Design review of the part built by this model. Coordinates are the model's own, in mm. Coordinates: 2 decimals unless noted, no trailing zeros. Loops run counter-clockwise (first coordinate to the right, second up) from the corner with the lowest first, then second, coordinate; pieces in that order, holes last.
Q1. Add section C-C on z = -18.5. Give the boundary of the cut face in (x, y), and give its area (3 significant figures).
Q2. Add section B-B on y = 0.65. Give the boundary of the cut face in (x, z).
Q3. Add section A-A on x = 1. Give the boundary of the cut face in (y, z), and give its area (3 significant figures).
Q4. For P1, Ø1.2, axis at x = 6, z = -18.5, coming from the +Y side, flat-tipped, find the tip position at first contact; note if it passes through.
Q5. Wall thickness on probe 1 along X at (y, z) = (1.1, -13.5); probe 2 along X at (y, z) = (1.35, -13); probe 3 along X at (y, z) = (1.2, -28): over which ranges is each line inside the solid? List them lowest first.
```python
from build123d import *

# Parameters (mm, degrees)
BOSS_EXTRUDE1_DEPTH = 2
CUT_EXTRUDE2_REACH  = 58.071
SKETCH8_R           = 0.75


with BuildPart() as part:
    # Sketch1 → Boss-Extrude1 (new body)
    with BuildSketch(Plane(origin=(0, 0, 0), x_dir=(1, 0, 0), z_dir=(0, 1, 0))):
        with BuildLine():
            Line((5, 0), (41, 0))
            ThreePointArc((41, 0), (44.535533906, 1.464466094), (46, 5))
            Line((46, 5), (46, 27))
            ThreePointArc((46, 27), (44.535533906, 30.535533906), (41, 32))
            Line((41, 32), (5, 32))
            ThreePointArc((5, 32), (1.464466094, 30.535533906), (0, 27))
            Line((0, 27), (0, 5))
            ThreePointArc((0, 5), (1.464466094, 1.464466094), (5, 0))
        make_face()
    extrude(amount=BOSS_EXTRUDE1_DEPTH)

    # Sketch8 → Cut-Extrude2 (cut, up to next)
    with BuildSketch(Plane(origin=(0, 2, 0), x_dir=(1, 0, 0), z_dir=(0, 1, 0)), mode=Mode.PRIVATE) as cut_extrude2_sk1:
        with Locations(Location((3.5, 16, 0), (0, 0, 270))):
            Circle(SKETCH8_R)
    cut_extrude2_tool1 = extrude(cut_extrude2_sk1.sketch, amount=-CUT_EXTRUDE2_REACH, mode=Mode.PRIVATE) & part.part
    # Sketch8 → Cut-Extrude2 (cut, up to next)
    with BuildSketch(Plane(origin=(0, 2, 0), x_dir=(1, 0, 0), z_dir=(0, 1, 0)), mode=Mode.PRIVATE) as cut_extrude2_sk2:
        with Locations(Location((6, 18.5, 0), (0, 0, 270))):
            Circle(SKETCH8_R)
    cut_extrude2_tool2 = extrude(cut_extrude2_sk2.sketch, amount=-CUT_EXTRUDE2_REACH, mode=Mode.PRIVATE) & part.part
    # Sketch8 → Cut-Extrude2 (cut, up to next)
    with BuildSketch(Plane(origin=(0, 2, 0), x_dir=(1, 0, 0), z_dir=(0, 1, 0)), mode=Mode.PRIVATE) as cut_extrude2_sk3:
        with Locations(Location((6, 13.5, 0), (0, 0, 270))):
            Circle(SKETCH8_R)
    cut_extrude2_tool3 = extrude(cut_extrude2_sk3.sketch, amount=-CUT_EXTRUDE2_REACH, mode=Mode.PRIVATE) & part.part
    # Sketch8 → Cut-Extrude2 (cut, up to next)
    with BuildSketch(Plane(origin=(0, 2, 0), x_dir=(1, 0, 0), z_dir=(0, 1, 0)), mode=Mode.PRIVATE) as cut_extrude2_sk4:
        with Locations(Location((1, 13.499992953, 0), (0, 0, 270))):
            Circle(SKETCH8_R)
    cut_extrude2_tool4 = extrude(cut_extrude2_sk4.sketch, amount=-CUT_EXTRUDE2_REACH, mode=Mode.PRIVATE) & part.part
    # Sketch8 → Cut-Extrude2 (cut, up to next)
    with BuildSketch(Plane(origin=(0, 2, 0), x_dir=(1, 0, 0), z_dir=(0, 1, 0)), mode=Mode.PRIVATE) as cut_extrude2_sk5:
        with Locations(Location((1, 18.499992953, 0), (0, 0, 270))):
            Circle(SKETCH8_R)
    cut_extrude2_tool5 = extrude(cut_extrude2_sk5.sketch, amount=-CUT_EXTRUDE2_REACH, mode=Mode.PRIVATE) & part.part
    add(cut_extrude2_tool1.solids().sort_by_distance((3.5, 2, -16))[0], mode=Mode.SUBTRACT)
    add(cut_extrude2_tool2.solids().sort_by_distance((6, 2, -18.5))[0], mode=Mode.SUBTRACT)
    add(cut_extrude2_tool3.solids().sort_by_distance((6, 2, -13.5))[0], mode=Mode.SUBTRACT)
    add(cut_extrude2_tool4.solids().sort_by_distance((1, 2, -13.499993))[0], mode=Mode.SUBTRACT)
    add(cut_extrude2_tool5.solids().sort_by_distance((1, 2, -18.499993))[0], mode=Mode.SUBTRACT)


solid = part.part
```
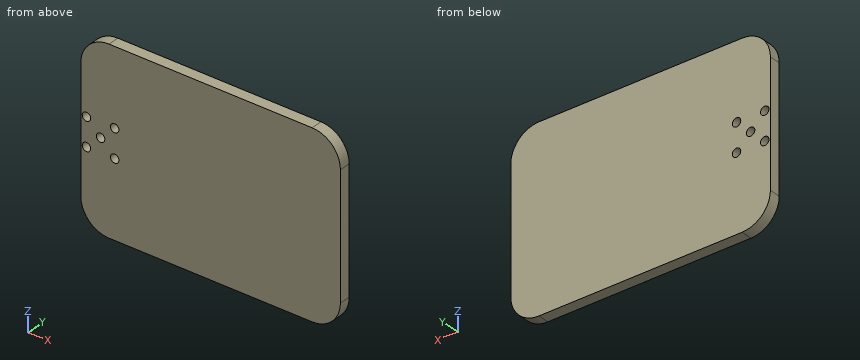
Entries:
1. outline: (0, 0) - (0.25, 0) - (0.25, 2) - (0, 2) - close; (1.75, 0) - (5.25, 0) - (5.25, 2) - (1.75, 2) - close; (6.75, 0) - (46, 0) - (46, 2) - (6.75, 2) - close
1. area: 86.0 mm2
2. outline: (0, -27) arc R5 ccw to (5, -32) - (41, -32) arc R5 ccw to (46, -27) - (46, -5) arc R5 ccw to (41, 0) - (5, 0) arc R5 ccw to (0, -5) - close; hole circle Ø1.5 at (1, -18.5); hole circle Ø1.5 at (1, -13.5); hole circle Ø1.5 at (3.5, -16); hole circle Ø1.5 at (6, -18.5); hole circle Ø1.5 at (6, -13.5)
3. outline: (0, -30) - (2, -30) - (2, -19.25) - (0, -19.25) - close; (0, -17.75) - (2, -17.75) - (2, -14.25) - (0, -14.25) - close; (0, -12.75) - (2, -12.75) - (2, -2) - (0, -2) - close
3. area: 50.0 mm2
4. P1: passes through
5. probe 1: x = 0 to 0.25, 1.75 to 5.25, 6.75 to 46
5. probe 2: x = 0 to 0.44, 1.56 to 5.44, 6.56 to 46
5. probe 3: x = 0.1 to 45.9
